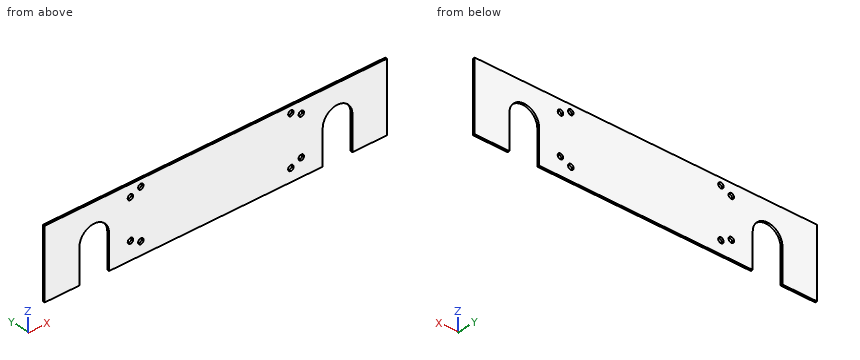
from build123d import *

# Parameters (mm, degrees)
SKETCH1_W            = 346
SKETCH1_H            = 2
BOSS_EXTRUDE1_DEPTH  = 70
M5_CLEARANCE_HOLE1_D = 5.5
CUT_EXTRUDE1_DEPTH   = 10


with BuildPart() as part:
    # Sketch1 → Boss-Extrude1 (new body)
    with BuildSketch(Plane.XY):
        Rectangle(SKETCH1_W, SKETCH1_H)
    extrude(amount=BOSS_EXTRUDE1_DEPTH)

    # M5 Clearance Hole1 (through all)
    with Locations(Plane(origin=(86.36, 1, 18), x_dir=(1, 0, 0), z_dir=(0, 1, 0))):
        with Locations((0, 0), (-10.5, 5), (0, -40), (-10.5, -45)):
            m5_clearance_hole1 = Hole(M5_CLEARANCE_HOLE1_D / 2)

    # Mirror1: M5 Clearance Hole1 across plane
    add(m5_clearance_hole1.mirror(Plane(origin=(0, 0, 0), x_dir=(0, 0, 1), z_dir=(1, 0, 0))), mode=Mode.SUBTRACT)

    # Sketch4 → Cut-Extrude1 (cut)
    with BuildSketch(Plane(origin=(0, 1, 0), x_dir=(1, 0, 0), z_dir=(0, 1, 0))):
        with BuildLine():
            Line((138, -35), (138, 0))
            Line((138, 0), (108, 0))
            Line((108, 0), (108, -35))
            ThreePointArc((108, -35), (123, -50), (138, -35))
        make_face()
        with BuildLine():
            Line((-108, -35), (-108, 0))
            Line((-108, 0), (-138, 0))
            Line((-138, 0), (-138, -35))
            ThreePointArc((-138, -35), (-123, -50), (-108, -35))
        make_face()
    extrude(amount=-CUT_EXTRUDE1_DEPTH, mode=Mode.SUBTRACT)


solid = part.part
Here's how the part is built. I have some questions about the finished solid (model axes, mm). Give positions to 0.01 mm unless a question says otherwise; leave off trailing zeros. Write each loop counter-clockwise with the first axis right and the second up, starting at its lowest first coordinate (ties: lowest second). Pieces come first, ordered by that corner, then holes. Notation, with made-up numbers: (1, 66) -> (5, 66) arc R19 cw to (5, 90) -> close; hole circle Ø11 at (14, -21.75). An arc over 180 degrees is marked (long way). Use one line per item in the form item = value. Start each with the question number.
1. Imagine slicing it at B-B on y = -0.1. State how many separate pieces and enclosed holes the cut face has, plus the area to 3 significant figures.
2. Imagine slicing it at C-C on x = -123. List the corners of the cut face in (y, z) for me.
3. Imagine slicing it at A-A on z = 24. List the corners of the cut face in (x, y) for me, plus the area to 3 significant figures.
4. If I drill on L1, parallel to Z at x = -75.86, y = -0.55; L2, parallel to Z at x = 86.36, y = 0.45; L3, parallel to X at y = -0.6, z = 5.5, over which ranges is the centre line in solid material (lowest first)?
Entries:
q1.separate_pieces = 1
q1.enclosed_holes = 8
q1.area = 21,200 mm²
q2.outline = (-1, 50) -> (1, 50) -> (1, 70) -> (-1, 70) -> close
q3.outline = (-173, -1) -> (-138, -1) -> (-138, 1) -> (-173, 1) -> close; (-108, -1) -> (108, -1) -> (108, 1) -> (-108, 1) -> close; (138, -1) -> (173, -1) -> (173, 1) -> (138, 1) -> close
q3.area = 572 mm²
q4.L1 = 0 to 10.25, 15.75 to 60.25, 65.75 to 70
q4.L2 = 0 to 15.25, 20.75 to 55.25, 60.75 to 70
q4.L3 = -173 to -138, -108 to 108, 138 to 173
